from build123d import *

# Parameters (mm, degrees)
SKIZZE1_W                       = 90
SKIZZE1_H                       = 50
AUFSATZ_LINEAR_AUSTRAGEN1_DEPTH = 0.4
SKIZZE3_R                       = 1.5
SCHNITT_LINEAR_AUSTRAGEN1_DEPTH = 1.4
SKIZZE18_R                      = 2.5
SKIZZE18_R_2                    = 1.5
AUFSATZ_LINEAR_AUSTRAGEN5_DEPTH = 1.6
SKIZZE22_R                      = 1.45
AUFSATZ_LINEAR_AUSTRAGEN7_DEPTH = 18
SKIZZE24_W                      = 4
SKIZZE24_H                      = 22.665276743
AUFSATZ_LINEAR_AUSTRAGEN8_DEPTH = 1.5
SKIZZE25_W                      = 0.4
SKIZZE25_H                      = 3.961895835
SCHNITT_LINEAR_AUSTRAGEN4_DEPTH = 91
SKIZZE26_R                      = 1.45
SCHNITT_LINEAR_AUSTRAGEN5_DEPTH = 1


with BuildPart() as part:
    # Skizze1 → Aufsatz-Linear austragen1 (new body)
    with BuildSketch(Plane.XY):
        Rectangle(SKIZZE1_W, SKIZZE1_H)
    extrude(amount=AUFSATZ_LINEAR_AUSTRAGEN1_DEPTH)

    # Skizze3 → Schnitt-Linear austragen1 (cut, through all)
    with BuildSketch(Plane.XY.offset(0.4)):
        with Locations((-26.9, 19.461895835)):
            Circle(SKIZZE3_R)
        with Locations((26.9, 19.461895835)):
            Circle(SKIZZE3_R)
        with Locations((26.9, -11.538104165)):
            Circle(SKIZZE3_R)
        with Locations((-26.9, -11.538104165)):
            Circle(SKIZZE3_R)
    extrude(amount=-SCHNITT_LINEAR_AUSTRAGEN1_DEPTH, mode=Mode.SUBTRACT)

    # Skizze18 → Aufsatz-Linear austragen5 (add)
    with BuildSketch(Plane.XY.offset(0.4)):
        with Locations((-26.9, 19.461895835)):
            Circle(SKIZZE18_R)
        with Locations((-26.9, 19.461895835)):
            Circle(SKIZZE18_R_2, mode=Mode.SUBTRACT)
        with Locations((26.9, 19.461895835)):
            Circle(SKIZZE18_R)
        with Locations((26.9, 19.461895835)):
            Circle(SKIZZE18_R_2, mode=Mode.SUBTRACT)
        with Locations((26.9, -11.538104165)):
            Circle(SKIZZE18_R)
        with Locations((26.9, -11.538104165)):
            Circle(SKIZZE18_R_2, mode=Mode.SUBTRACT)
        with Locations((-26.9, -11.538104165)):
            Circle(SKIZZE18_R)
        with Locations((-26.9, -11.538104165)):
            Circle(SKIZZE18_R_2, mode=Mode.SUBTRACT)
    extrude(amount=AUFSATZ_LINEAR_AUSTRAGEN5_DEPTH)

    # Skizze22 → Aufsatz-Linear austragen7 (add)
    with BuildSketch(Plane.XY.offset(0.4)):
        Polygon((30.75, -15.038104165), (0, -15.038104165), (-30.75, -15.038104165), (-30.75, -11.965150571), (-34.75, -11.965150571), (-34.75, -19.038104165), (0, -19.038104165), (34.75, -19.038104165), (34.75, -11.965150571), (30.75, -11.965150571), align=None)
        with Locations((32.75, -17.038104165)):
            Circle(SKIZZE22_R, mode=Mode.SUBTRACT)
        with Locations((6.45, -17.038104165)):
            Circle(SKIZZE22_R, mode=Mode.SUBTRACT)
        with Locations((-6.45, -17.038104165)):
            Circle(SKIZZE22_R, mode=Mode.SUBTRACT)
        with Locations((-32.75, -17.038104165)):
            Circle(SKIZZE22_R, mode=Mode.SUBTRACT)
        Polygon((34.75, 15.223665498), (34.75, 18.83332796), (30.75, 18.83332796), (30.75, 15.223665498), (30.75, 10.700126172), (34.75, 10.700126172), align=None)
        with Locations((32.75, 12.961895835)):
            Circle(SKIZZE22_R, mode=Mode.SUBTRACT)
        Polygon((-30.75, 18.83332796), (-30.75, 15.223665498), (-30.75, 10.700126172), (-34.75, 10.700126172), (-34.75, 15.223665498), (-34.75, 18.83332796), align=None)
        with Locations((-32.75, 12.961895835)):
            Circle(SKIZZE22_R, mode=Mode.SUBTRACT)
    extrude(amount=AUFSATZ_LINEAR_AUSTRAGEN7_DEPTH)

    # Skizze24 → Aufsatz-Linear austragen8 (add)
    with BuildSketch(Plane.XY.offset(0.4)):
        with Locations((-32.75, -0.632512199)):
            Rectangle(SKIZZE24_W, SKIZZE24_H)
        with Locations((32.75, -0.632512199)):
            Rectangle(SKIZZE24_W, SKIZZE24_H)
    extrude(amount=AUFSATZ_LINEAR_AUSTRAGEN8_DEPTH)

    # Skizze25 → Schnitt-Linear austragen4 (cut, through all)
    with BuildSketch(Plane(origin=(45, 0, 0), x_dir=(0, 0, -1), z_dir=(1, 0, 0))):
        with Locations((-0.2, -23.019052083)):
            Rectangle(SKIZZE25_W, SKIZZE25_H)
    extrude(amount=-SCHNITT_LINEAR_AUSTRAGEN4_DEPTH, mode=Mode.SUBTRACT)

    # Skizze26 → Schnitt-Linear austragen5 (cut)
    with BuildSketch(Plane(origin=(0, 0, 0), x_dir=(-1, 0, 0), z_dir=(0, 0, -1))):
        with Locations((-40.5, -16.7)):
            Circle(SKIZZE26_R)
        with Locations((-40.5, 21.3)):
            Circle(SKIZZE26_R)
        with Locations((40.5, -16.7)):
            Circle(SKIZZE26_R)
        with Locations((40.5, 21.3)):
            Circle(SKIZZE26_R)
    extrude(amount=-SCHNITT_LINEAR_AUSTRAGEN5_DEPTH, mode=Mode.SUBTRACT)


solid = part.part
Here's how the part is built. I have some questions about the finished solid (model axes, mm). A direction names the side the tool comes from. Coordinates: 2 decimals unless noted, no trailing zeros. Loops run counter-clockwise (first coordinate to the right, second up) from the corner with the lowest first, then second, coordinate; pieces in that order, holes last.
1. Imagine slicing it at B-B, the plane x = -6.45. Please give me the cut outline in (y, z).
2. Imagine slicing it at A-A, the plane x = -26.9. Please give me the cut outline in (y, z).
3. I need wall thicknesses on L1, parallel to Y at x = -26.9, z = 1.3; L2, parallel to X at y = -15, z = 11.25; L3, parallel to Y at x = 30, z = 7.25. Which ranges of each line are inside material? Lowest first, please.
4. Imagine slicing it at D-D, the plane x = -40.5. Please give me the cut outline in (y, z).
5. If we mould it in two halves opening along Y, with no side actions, what happens to faces 1 (the flat face through (-33, 16, 18.4)), 2 (the flat face through (-33, 10.7, 10)), 3 (the flat face through (33, 18.833, 9))? For each: pulls with the +Y half, pulls with the -Y half, needs draft (parallel to the pull), parting line crosses it, or undercut.
6. Imagine slicing it at C-C, the plane z = 8.25. Count the separate pieces of the cut face and the enclosed holes in it, and give its area (3 significant figures).
7. For P1, Ø2, axis at x = -33.5, y = 4, coming from the +Z side; P2, Ø4, axis at x = -26.9, y = -11.54, coming from the -Z side; P3, Ø5, axis at y = -16, z = 13.5, coming from the +X side; P4, Ø2, axis at x = -33, z = 10.5, coming from the +Y side, each with a flat end and sliding along its axis, tell me the tip position at first contact or that it passes through.
8. For faces 4 (the flat face through (30.75, 6, 1)), 5 (the flat face through (0, -19.038, 9)), 6 (the cylindrical face through (-25.556, -9.43, 1.189)), 7 (the cylindrical face through (-39.05, -16.64, 0.2)), which set-ups out of +Z, -Z, +X, -X, +Y, -Y let a thin tool reach every point of the face, with its end or its side?
Taken from the geometry:
1. outline: (-21.04, 0) - (25, 0) - (25, 0.4) - (-15.04, 0.4) - (-15.04, 18.4) - (-15.59, 18.4) - (-15.59, 0.4) - (-18.49, 0.4) - (-18.49, 18.4) - (-19.04, 18.4) - (-19.04, 0.4) - (-21.04, 0.4) - close
2. outline: (-21.04, 0) - (-13.04, 0) - (-13.04, 2) - (-14.04, 2) - (-14.04, 0.4) - (-15.04, 0.4) - (-15.04, 18.4) - (-19.04, 18.4) - (-19.04, 0.4) - (-21.04, 0.4) - close; (-10.04, 0) - (17.96, 0) - (17.96, 2) - (16.96, 2) - (16.96, 0.4) - (-9.04, 0.4) - (-9.04, 2) - (-10.04, 2) - close; (20.96, 0) - (25, 0) - (25, 0.4) - (21.96, 0.4) - (21.96, 2) - (20.96, 2) - close
3. L1: y = -19.04 to -15.04, -14.04 to -13.04, -10.04 to -9.04, 16.96 to 17.96, 20.96 to 21.96
3. L2: x = -34.75 to -30.75, 30.75 to 34.75
3. L3: y = -19.04 to -15.04
4. outline: (-21.04, 0) - (-18.15, 0) - (-18.15, 0.4) - (-21.04, 0.4) - close; (-15.25, 0) - (19.85, 0) - (19.85, 0.4) - (-15.25, 0.4) - close; (22.75, 0) - (25, 0) - (25, 0.4) - (22.75, 0.4) - close
5. face 1: needs draft
5. face 2: undercut
5. face 3: pulls with the +Y half
6. separate pieces: 3
6. enclosed holes: 6
6. area: 328 mm2
7. P1: stops at z = 1.9
7. P2: stops at z = 0
7. P3: stops at x = 34.75
7. P4: stops at y = 18.83
8. face 4: +Z, +Y
8. face 5: +Z, +X, -X, -Y
8. face 6: +Z
8. face 7: +Z, -Z
